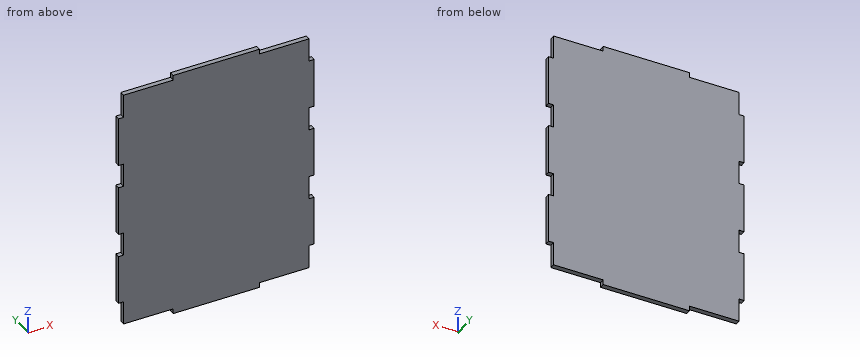
Autodesk Inventor part; units mm, degrees
ref_plane "YZ Plane" through (0, 0, 0) normal (1, 0, 0) x (0, 1, 0)
ref_plane "XZ Plane" through (0, 0, 0) normal (0, 1, 0) x (-1, 0, 0)
ref_plane "XY Plane" through (0, 0, 0) normal (0, 0, 1) x (1, 0, 0)
sketch "Sketch1" plane through (0, 0, 0) normal (0, 1, 0) x (-1, 0, 0)
  line L0 (0, 0) -> (187, 0)
  line L1 (187, 0) -> (187, -245)
  line L2 (187, -245) -> (0, -245)
  line L3 (0, -245) -> (0, 0)
  dimension "d0" = 245
  dimension "d1" = 187
extrude "Extrusion1" add sketch "Sketch1" along normal blind 5
sketch "Sketch2" plane through (0, 5, 0) normal (0, 1, 0) x (1, 0, 0)
  line L0 (-187, 0) -> (0, 0)
  line L1 (0, 0) -> (0, 245)
  line L2 (0, 245) -> (-187, 245)
  line L3 (-187, 245) -> (-187, 0)
  line L4 (-187, 221.25) -> (-192, 221.25)
  line L5 (-192, 221.25) -> (-192, 171.25)
  line L6 (-192, 171.25) -> (-187, 171.25)
  line L7 (-187, 171.25) -> (-187, 221.25)
  line L8 (-192, 147.5) -> (-187, 147.5)
  line L9 (-187, 147.5) -> (-187, 97.5)
  line L10 (-187, 97.5) -> (-192, 97.5)
  line L11 (-192, 97.5) -> (-192, 147.5)
  line L12 (-192, 73.75) -> (-187, 73.75)
  line L13 (-187, 73.75) -> (-187, 23.75)
  line L14 (-187, 23.75) -> (-192, 23.75)
  line L15 (-192, 23.75) -> (-192, 73.75)
  line L16 (5, 221.25) -> (0, 221.25)
  line L17 (0, 221.25) -> (0, 171.25)
  line L18 (0, 171.25) -> (5, 171.25)
  line L19 (5, 171.25) -> (5, 221.25)
  line L20 (0, 147.5) -> (5, 147.5)
  line L21 (5, 147.5) -> (5, 97.5)
  line L22 (5, 97.5) -> (0, 97.5)
  line L23 (0, 97.5) -> (0, 147.5)
  line L24 (0, 73.75) -> (5, 73.75)
  line L25 (5, 73.75) -> (5, 23.75)
  line L26 (5, 23.75) -> (0, 23.75)
  line L27 (0, 23.75) -> (0, 73.75)
  line L28 (-137, 250) -> (-50, 250)
  line L29 (-50, 250) -> (-50, 245)
  line L30 (-50, 245) -> (-137, 245)
  line L31 (-137, 245) -> (-137, 250)
  line L32 (-137, 0) -> (-50, 0)
  line L33 (-50, 0) -> (-50, -5)
  line L34 (-50, -5) -> (-137, -5)
  line L35 (-137, -5) -> (-137, 0)
  point P0 (-50, 0)
  dimension "d4" = 5
  dimension "d5" = 50
  dimension "d6" = 50
  dimension "d7" = 50
  dimension "d8" = 5
  dimension "d9" = 5
  dimension "d10" = 23.75
  dimension "d11" = 23.75
  dimension "d12" = 23.75
  dimension "d13" = 5
  dimension "d14" = 50
  dimension "d15" = 50
  dimension "d16" = 50
  dimension "d17" = 5
  dimension "d18" = 5
  dimension "d19" = 23.75
  dimension "d20" = 23.75
  dimension "d21" = 23.75
  dimension "d22" = 5
  dimension "d23" = 50
  dimension "d24" = 50
  dimension "d25" = 5
  dimension "d26" = 50
  dimension "d27" = 50
extrude "Extrusion2" add sketch "Sketch2" against normal blind 5 contours L0 L33 L34 L35 | L14 L15 L12 L3 | L10 L11 L8 L3 | L1 L24 L25 L26 | L6 L5 L4 L3 | L1 L20 L21 L22 | L1 L16 L19 L18 | L31 L28 L29 L2
properties part number "Placa de abajo"
Design review of the part built by this model. Coordinates are the model's own, in mm. Round coordinates to 2 decimals unless told otherwise and drop trailing zeros. Write each loop counter-clockwise with the first axis right and the second up, starting at its lowest first coordinate (ties: lowest second). Pieces come first, ordered by that corner, then holes.
Item 1: Consider section B-B on x = -12.5. Give the boundary of the cut face in (y, z), and give its area (4 significant figures).
Item 2: Wall thickness on L1, parallel to X at y = 2.95, z = -226; L2, parallel to Z at x = -48.5, y = 3.7: over which ranges is each line inside the solid? List them lowest first.
Item 3: For pin 1 Ø1.5 at (x, y) = (-188.5, 3) entering from -Z; pin 2 Ø2.5 at (y, z) = (3, -238.5) entering from +X; pin 3 Ø1.5 at (x, y) = (1.5, 3) entering from +Z, all flat-tipped, find the tip position at first contact; note any pin that passes through.
Item 4: Consider section A-A on z = -159. Give the boundary of the cut face in (x, y), and give its area (3 significant figures).
Check values:
1. outline: (0, -245) - (5, -245) - (5, 0) - (0, 0) - close
1. area: 1,225 mm2
2. L1: x = -187 to 0
2. L2: z = -245 to 0
3. pin 1: stops at z = -221.25
3. pin 2: stops at x = 0
3. pin 3: stops at z = -23.75
4. outline: (-187, 0) - (0, 0) - (0, 5) - (-187, 5) - close
4. area: 935 mm2
